Geometry: final body of the model. Coordinates: model frame, mm. Face numbers are marked on the shaded views. A direction names the side the tool comes from. Coordinates: 2 decimals unless noted, no trailing zeros. Order: outer loops, then holes, each group sorted by start corner. A loop starts at its lowest first (then second) coordinate and runs counter-clockwise, first axis right, second up. Notation, with made-up numbers: (10.5, 38.25) - (59.5, 38.25) arc R13 ccw to (59.5, 54.25) - close; hole circle Ø6 at (40.25, 1.5). An arc over 180 degrees is marked (long way). Use a Markdown table: item, result. Add a question column.
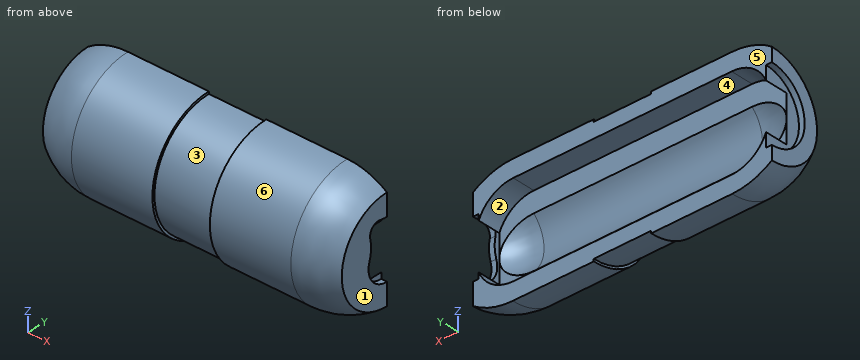
```python
from build123d import *

# Parameters (mm, degrees)
F2_ANGLE  = 180
F4_DEPTH  = 2.54
F6_W      = 6.35
F6_H      = 0.508
F9_DEPTH  = 2.54
F10_W     = 2.54
F10_H     = 11.1908745342
F11_DEPTH = 25.4
F13_DEPTH = 0.635
F15_DEPTH = 0.635
F17_DEPTH = 0.635
F18_R     = 4.064
F19_DEPTH = 0.635
F21_DEPTH = 2.54


with BuildPart() as f2:
    # F0 (on Front) → F2 (revolve)
    with BuildSketch(Plane.XZ):
        with BuildLine():
            ThreePointArc((19.05, 2.54), (16.2382381507, 5.7781856359), (12.1229678072, 6.985))
            Line((12.1229678072, 6.985), (-12.1229678072, 6.985))
            ThreePointArc((-12.1229678072, 6.985), (-16.2382381507, 5.7781856359), (-19.05, 2.54))
            Line((-19.05, 2.54), (-15.875, 2.54))
            ThreePointArc((-15.875, 2.54), (-14.0730463142, 3.4841389426), (-12.065, 3.81))
            Line((-12.065, 3.81), (12.065, 3.81))
            ThreePointArc((12.065, 3.81), (14.0730463142, 3.4841389426), (15.875, 2.54))
            Line((15.875, 2.54), (19.05, 2.54))
        make_face()
    revolve(axis=Axis((-1.6419366002, 0, 0), (1, 0, 0)), revolution_arc=F2_ANGLE)

    # F3 (on face) → F4 (cut)
    with BuildSketch(Plane(origin=(0, 0, 0), x_dir=(-1, 0, 0), z_dir=(0, 1, 0))):
        with BuildLine():
            ThreePointArc((15.875, -2.54), (14.0730463142, -3.4841389426), (12.065, -3.81))
            Line((12.065, -3.81), (-12.065, -3.81))
            ThreePointArc((-12.065, -3.81), (-14.0730463142, -3.4841389426), (-15.875, -2.54))
            ThreePointArc((-15.875, -2.54), (-14.3545250599, -4.3867875899), (-12.065, -5.08))
            Line((-12.065, -5.08), (12.065, -5.08))
            ThreePointArc((12.065, -5.08), (14.3531088493, -4.384663274), (15.875, -2.54))
        make_face()
        with BuildLine():
            ThreePointArc((15.875, 2.54), (14.3531088493, 4.384663274), (12.065, 5.08))
            Line((12.065, 5.08), (-12.065, 5.08))
            ThreePointArc((-12.065, 5.08), (-14.3545250599, 4.3867875899), (-15.875, 2.54))
            ThreePointArc((-15.875, 2.54), (-14.0730463142, 3.4841389426), (-12.065, 3.81))
            Line((-12.065, 3.81), (12.065, 3.81))
            ThreePointArc((12.065, 3.81), (14.0730463142, 3.4841389426), (15.875, 2.54))
        make_face()
    extrude(amount=-F4_DEPTH, mode=Mode.SUBTRACT)

    # F6 (on face) → F7 (revolve, cut)
    with BuildSketch(Plane(origin=(0, 0, 0), x_dir=(-1, 0, 0), z_dir=(0, 1, 0))):
        with Locations((0, 6.985)):
            Rectangle(F6_W, F6_H)
    revolve(axis=Axis((-0.6197560579, 0, 0), (-1, 0, 0)), mode=Mode.SUBTRACT)

    # F8 (on face) → F9 (cut)
    with BuildSketch(Plane(origin=(0, -2.54, 0), x_dir=(-1, 0, 0), z_dir=(0, 1, 0))):
        with BuildLine():
            Line((12.065, -3.302), (-12.065, -3.302))
            ThreePointArc((-12.065, -3.302), (-14.0964974368, -2.8562435921), (-15.875, -1.778))
            Line((-15.875, -1.778), (-15.875, -2.54))
            ThreePointArc((-15.875, -2.54), (-14.0730463142, -3.4841389426), (-12.065, -3.81))
            Line((-12.065, -3.81), (12.065, -3.81))
            ThreePointArc((12.065, -3.81), (14.0730463142, -3.4841389426), (15.875, -2.54))
            Line((15.875, -2.54), (15.875, -1.778))
            ThreePointArc((15.875, -1.778), (14.1167477915, -2.9068694788), (12.065, -3.302))
        make_face()
        with BuildLine():
            ThreePointArc((15.875, 2.54), (14.0730463142, 3.4841389426), (12.065, 3.81))
            Line((12.065, 3.81), (-12.065, 3.81))
            ThreePointArc((-12.065, 3.81), (-14.0730463142, 3.4841389426), (-15.875, 2.54))
            Line((-15.875, 2.54), (-15.875, 1.778))
            ThreePointArc((-15.875, 1.778), (-14.0964974368, 2.8562435921), (-12.065, 3.302))
            Line((-12.065, 3.302), (12.065, 3.302))
            ThreePointArc((12.065, 3.302), (14.1167477915, 2.9068694788), (15.875, 1.778))
            Line((15.875, 1.778), (15.875, 2.54))
        make_face()
    extrude(amount=F9_DEPTH, mode=Mode.SUBTRACT)

    # F10 (on face) → F11 (cut)
    with BuildSketch(Plane(origin=(0, 0, 0), x_dir=(-1, 0, 0), z_dir=(0, 1, 0))):
        with Locations((-17.78, 0)):
            Rectangle(F10_W, F10_H)
        with Locations((17.78, 0)):
            Rectangle(F10_W, F10_H)
    extrude(amount=-F11_DEPTH, mode=Mode.SUBTRACT)

    # F12 (on face) → F13 (join, through all)
    with BuildSketch(Plane.YZ.offset(16.51)):
        with BuildLine():
            Line((0, -2.54), (0, 2.54))
            ThreePointArc((0, 2.54), (-2.54, 0), (0, -2.54))
        make_face()
    extrude(amount=-F13_DEPTH)

    # F14 (on face) → F15 (cut, through all)
    with BuildSketch(Plane.YZ.offset(16.51)):
        with BuildLine():
            ThreePointArc((-2.0707510052, 2.0194225538), (-1.9696309355, 0.9047357394), (-2.1717097382, -0.1961348798))
            ThreePointArc((-2.1717097382, -0.1961348798), (0.0006908158, -3.195908418), (2.1712779452, -0.1948224543))
            ThreePointArc((2.1712779452, -0.1948224543), (1.9685414869, 0.9057599903), (2.0689058267, 2.0203499545))
            ThreePointArc((2.0689058267, 2.0203499545), (1.7968430427, 2.9874721132), (0.8360337914, 3.2810517634))
            ThreePointArc((0.8360337914, 3.2810517634), (4.14538e-05, 3.1959085075), (-0.8358696943, 3.281845199))
            ThreePointArc((-0.8358696943, 3.281845199), (-1.7984885251, 2.9882815567), (-2.0707510052, 2.0194225538))
        make_face()
    extrude(amount=-F15_DEPTH, mode=Mode.SUBTRACT)

    # F16 (on face) → F17 (join, through all)
    with BuildSketch(Plane(origin=(-16.51, 0, 0), x_dir=(0, -1, 0), z_dir=(-1, 0, 0))):
        with BuildLine():
            Line((0, 2.54), (0, -2.54))
            ThreePointArc((0, -2.54), (2.54, 0), (0, 2.54))
        make_face()
    extrude(amount=-F17_DEPTH)

    # F18 (on face) → F19 (cut, through all)
    with BuildSketch(Plane(origin=(-16.51, 0, 0), x_dir=(0, -1, 0), z_dir=(-1, 0, 0))):
        Circle(F18_R)
    extrude(amount=-F19_DEPTH, mode=Mode.SUBTRACT)

    # F20 (on face) → F21 (cut, through all)
    with BuildSketch(Plane(origin=(0, -2.54, 0), x_dir=(-1, 0, 0), z_dir=(0, 1, 0))):
        with BuildLine():
            Line((12.0565390969, 5.08), (-12.065, 5.08))
            ThreePointArc((-12.065, 5.08), (-14.3545250599, 4.3867875899), (-15.875, 2.54))
            Line((-15.875, 2.54), (-15.875, -2.54))
            ThreePointArc((-15.875, -2.54), (-14.3545250599, -4.3867875899), (-12.065, -5.08))
            Line((-12.065, -5.08), (12.056537613, -5.0800086453))
            ThreePointArc((12.056537613, -5.0800086453), (14.3495870824, -4.3870085201), (15.875, -2.54))
            Line((15.875, -2.54), (15.875, 2.54))
            ThreePointArc((15.875, 2.54), (14.3531088493, 4.384663274), (12.065, 5.08))
            Line((12.065, 5.08), (12.0565390969, 5.08))
        make_face()
    extrude(amount=F21_DEPTH, mode=Mode.SUBTRACT)


solid = f2.part
```
1) Ray query, line 1 along Z through (x, y) = (10, -0.25); line 2 along Z through (x, y) = (-12, -2.5); line 3 along Z through (x, y) = (-12, -5.25). Return the intervals inside material, ascending.
2) Section A-A (x = -1.5). Return loops of the section in (y, z).
3) Section B-B (x = 5). Return loops of the section in (y, z) (3 decimals).
4) Draft query along Z for the marked faces 4, 5 and 6. Return one class per face: pulls with the +Z half, pulls with the -Z half, needs draft (parallel to the pull), parting line crosses it, or undercut.
5) Pin query (flat end, axial travel): pin 1 (1.5 mm diameter, centred on x = 7, z = 3, fed in from +Y); pin 2 (1.3 mm diameter, centred on x = -0.5, y = -1.5, fed in from -Z); pin 3 (0.7 mm diameter, centred on y = -2, z = 1, fed in from -X) (3 decimals). Return the tip coordinate at first contact, or that it passes through.
6) Set-up query: the marked faces 1, 2 and 3. Return all of +Z, -Z, +X, -X, +Y, -Y with unobstructed straight access to the full face (end or side cutting, diameter ignored); none if empty.
Values follow:
| question | item | result |
|---|---|---|
| 1 | line 1 | z = -6.98 to -5.08, 5.08 to 6.98 |
| 1 | line 2 | z = -6.52 to -5.08, 5.08 to 6.52 |
| 1 | line 3 | z = -4.61 to 4.61 |
| 2 | outline | (-2.54, -5.08) - (-2.54, -2.84) arc R3.81 cw to (-2.54, 2.84) - (-2.54, 5.08) - (0, 5.08) - (0, 6.73) arc R6.73 ccw to (0, -6.73) - (0, -5.08) - close |
| 3 | outline | (-2.54, -5.08) - (-2.54, -2.84) arc R3.81 cw to (-2.54, 2.84) - (-2.54, 5.08) - (0, 5.08) - (0, 6.985) arc R6.985 ccw to (0, -6.985) - (0, -5.08) - close |
| 4 | face 4 | undercut |
| 4 | face 5 | needs draft |
| 4 | face 6 | parting line crosses it |
| 5 | pin 1 | stops at y = -2.54 |
| 5 | pin 2 | stops at z = -6.68 |
| 5 | pin 3 | stops at x = 15.875 |
| 6 | face 1 | +Z, -Z, +X, +Y, -Y |
| 6 | face 2 | +Y |
| 6 | face 3 | -Y |
